Solid Edge part; units mm, degrees
sketch "Sketch1" plane through (0, 0, 0) normal (0, 0, 1) x (1, 0, 0)
  circle A0 centre (-13.8, 35.3) radius 2.2
  circle A1 centre (-13.8, 4.7) radius 2.2
  circle A2 centre (13.8, 4.7) radius 2.2
  circle A3 centre (13.8, 35.3) radius 2.2
  line L0 (-20, -1.5) -> (20, -1.5)
  line L1 (20, -1.5) -> (20, 41.5)
  line L2 (20, 41.5) -> (-20, 41.5)
  line L3 (-20, 41.5) -> (-20, -1.5)
  dimension "D1" = 20
  dimension "D2" = 20
  dimension "D3" = 13.8
extrude "Protrusion1" add sketch "Sketch1" against normal blind 10
sketch "Sketch2" plane through (0, 0, 0) normal (1, 0, 0) x (0, 1, 0)
  line L0 (3.9, -7.35) -> (8.9, -7.35)
  line L1 (3.9, -7.35) -> (3.6, -7.35)
  line L2 (3.6, -7.35) -> (3.6, -5.1123)
  line L3 (2.721, -5.1123) -> (3.6, -5.1123)
  line L4 (2.721, -5.1123) -> (-1.0103, -5.1123)
  line L5 (-1.0103, -5.1123) -> (-1.0103, -3.9681)
  line L6 (-1.0103, -2.774) -> (-1.0103, -3.9681)
  line L7 (-12.5526, -2.774) -> (-1.0103, -2.774)
  line L8 (-12.5526, 0) -> (-12.5526, -2.774)
  line L9 (39.4373, 0) -> (-12.5526, 0)
  line L10 (39.4373, -5.1123) -> (39.4373, 0)
  line L11 (38.3428, -5.1123) -> (39.4373, -5.1123)
  line L12 (34.6612, -5.1123) -> (38.3428, -5.1123)
  line L13 (34.4, -5.1123) -> (34.6612, -5.1123)
  line L14 (34.4, -7.3511) -> (34.4, -5.1123)
  line L15 (29.1, -7.3511) -> (34.4, -7.3511)
  line L16 (29.1, -7.3511) -> (28.8, -7.3511)
  line L17 (28.8, -7.3511) -> (28.8, -5.1123)
  line L18 (24.4125, -5.1123) -> (28.8, -5.1123)
  line L19 (24.4125, -2.774) -> (24.4125, -5.1123)
  line L20 (13.517, -2.774) -> (24.4125, -2.774)
  line L21 (13.517, -5.1123) -> (13.517, -2.774)
  line L22 (10.0842, -5.1123) -> (13.517, -5.1123)
  line L23 (9.2, -5.1123) -> (10.0842, -5.1123)
  line L24 (9.2, -7.35) -> (9.2, -5.1123)
  line L25 (8.9, -7.35) -> (9.2, -7.35)
  dimension "D1" = 3.9
  dimension "D2" = 3.9
  dimension "D3" = 8.9
revolve "RevolvedCutout1" cut sketch "Sketch2" angle 360 about axis through (0, -60, 0) along (0, 1, 0)
sketch "Sketch3" plane through (0, -1.5, -5) normal (0, -1, 0) x (1, 0, 0)
  line L0 (-23.1839, 5) -> (21.8988, 5)
  line L1 (21.8988, 5) -> (21.8988, 3.5)
  line L2 (21.8988, 3.5) -> (-23.1839, 3.5)
  line L3 (-23.1839, 3.5) -> (-23.1839, 5)
  dimension "D1" = 23.1839
extrude "ExtrudedCutout_2" cut sketch "Sketch3" against normal blind 318.8634
Design review of the part built by this model. Coordinates are the model's own, in mm. A direction names the side the tool comes from. Give positions to 0.01 mm unless a question says otherwise; leave off trailing zeros. Loops run counter-clockwise (first coordinate to the right, second up) from the corner with the lowest first, then second, coordinate; pieces in that order, holes last. Notation, with made-up numbers: M 34,-10 L 54,-10 A28 cw 54,23 Z; hole C 3,70 d3. An arc over 180 degrees is marked long. Return JSON: item names as keys, results as strings. Group by question number.
Item 1: We need section C-C (z = -9.5). Give the boundary of the cut face in (x, y), and give its area (3 significant figures).
Item 2: We need section B-B (y = 35.3). Give the boundary of the cut face in (x, z).
Item 3: For probe 1 along Y at (x, z) = (13.8, -4); probe 2 along Y at (x, z) = (-6, -3); probe 3 along X at (y, z) = (26, -3.5), list the stretches that pass through material, from the lowest coordinate up.
Item 4: Tool access review of faces 1 (the flat face through (0, 28.8, -6)), 2 (the cylindrical face through (13.51, 37.48, -5.69)): name each direction out of +Z, -Z, +X, -X, +Y, -Y from which nothing blocks a thin tool from reaching the whole face with its end or side.
Item 5: We need section D-D (z = -4). Give the number of separate pieces and of enclosed holes in the cut face, and give its area (3 significant figures).
Item 6: We need section A-A (x = 13.8). Give the boundary of the cut face in (y, z).
Item 7: Insertion check: pin 1 Ø4 at (x, y) = (-15, 4) entering from -Z. The pin has a flat end and moves straight along its axis. Give the tip position at first contact, or say it passes through.
Item 8: Mouldability with a two-part tool opening along X and no side actions: class faces 3 (the flat face through (-20, 20, -6)), 4 (the flat face through (0, -1.5, -6)), 5 (the cylindrical face through (0.039, 19.041, -2.774)) as released by +X, released by -X, zero draft, split by the parting line, or undercut.
Output:
{
 "1": {"outline": "M -20,-1.5 L 20,-1.5 L 20,41.5 L -20,41.5 Z; hole C -13.8,4.7 d4.4; hole C -13.8,35.3 d4.4; hole C 13.8,4.7 d4.4; hole C 13.8,35.3 d4.4", "area": "1,660 mm^2"},
 "2": {"outline": "M -20,-10 L -16,-10 L -16,-1.5 L -20,-1.5 Z; M -11.6,-10 L 11.6,-10 L 11.6,-1.5 L 4.89,-1.5 A5.11 cw -4.89,-1.5 L -11.6,-1.5 Z; M 16,-10 L 20,-10 L 20,-1.5 L 16,-1.5 Z"},
 "3": {"probe 1": "y = -1.5 to 2.5, 6.9 to 33.1, 37.5 to 41.5", "probe 2": "y = -1.5 to 3.6, 9.2 to 28.8, 34.4 to 41.5", "probe 3": "x = -20 to -3.73, 3.73 to 20"},
 "4": {"face 1": "+Z", "face 2": "+Z, -Z"},
 "5": {"separate pieces": "1", "enclosed holes": "6", "area": "1,400 mm^2"},
 "6": {"outline": "M -1.5,-10 L 2.5,-10 L 2.5,-1.5 L -1.5,-1.5 Z; M 6.9,-10 L 33.1,-10 L 33.1,-1.5 L 6.9,-1.5 Z; M 37.5,-10 L 41.5,-10 L 41.5,-1.5 L 37.5,-1.5 Z"},
 "7": {"pin 1": "stops at z = -10"},
 "8": {"face 3": "released by -X", "face 4": "zero draft", "face 5": "undercut"}
}
